```python
from build123d import *

# Parameters (mm, degrees)
BOSS_EXTRUDE1_DEPTH = 38.1


with BuildPart() as part:
    # Sketch1 → Boss-Extrude1 (new body)
    # profile 1 of 2: a face of its own
    with BuildSketch(Plane(origin=(0, 0, 0), x_dir=(1, 0, 0), z_dir=(0, 1, 0))):
        Polygon((0, 254), (0, 274), (-60.8, 250.891892714), (-60.8, 184.972107286), (-15, 175.951549331), (-15, 127), (0, 127), (0, 183.18932995), (-50.8, 193.194664975), (-50.8, 243.994664975), align=None)
    # profile 2 of 2: a face of its own
    with BuildSketch(Plane(origin=(0, 0, 0), x_dir=(1, 0, 0), z_dir=(0, 1, 0))):
        Polygon((99.289745962, 271.5), (107.95, 271.5), (107.95, 274), (0, 274), (0, 254), (107.95, 254), (107.95, 256.5), align=None)
        Polygon((85.629491924, 256.5), (94.289745962, 271.5), (102.95, 256.5), align=None, mode=Mode.SUBTRACT)
        Polygon((58.308983849, 256.5), (66.969237886, 271.5), (75.629491924, 256.5), align=None, mode=Mode.SUBTRACT)
        Polygon((89.289745962, 271.5), (80.629491924, 256.5), (71.969237886, 271.5), align=None, mode=Mode.SUBTRACT)
        Polygon((30.988475773, 256.5), (39.648729811, 271.5), (48.308983849, 256.5), align=None, mode=Mode.SUBTRACT)
        Polygon((61.969237886, 271.5), (53.308983849, 256.5), (44.648729811, 271.5), align=None, mode=Mode.SUBTRACT)
        Polygon((34.648729811, 271.5), (25.988475773, 256.5), (17.328221735, 271.5), align=None, mode=Mode.SUBTRACT)
        Polygon((12.328221735, 271.5), (20.988475773, 256.5), (3.667967697, 256.5), align=None, mode=Mode.SUBTRACT)
    extrude(amount=BOSS_EXTRUDE1_DEPTH)

    # Mirror1: part across plane


with BuildPart() as part_1:
    add(part.part)
    add(part.part.mirror(Plane(origin=(0, 38.1, -127), x_dir=(1, 0, 0), z_dir=(0, 0, -1))))

    # Mirror2: part across plane


with BuildPart() as part_2:
    add(part_1.part)
    add(part_1.part.mirror(Plane(origin=(107.95, 38.1, -254), x_dir=(0, 0, 1), z_dir=(-1, 0, 0))))


solid = part_2.part
```
Part model, mm, in its own coordinate system. A direction names the side the tool comes from. Coordinates: 2 decimals unless noted, no trailing zeros. Loops run counter-clockwise (first coordinate to the right, second up) from the corner with the lowest first, then second, coordinate; pieces in that order, holes last. Notation, with made-up numbers: (44, 51.5) - (91, 51.5) arc R6 cw to (91, 56.5) - close; hole circle Ø1 at (2, -34). An arc over 180 degrees is marked (long way). Write item = value, one per line. Start each with the question number.
Item 1: Cut at A-A, the plane z = -228.5. Give the cut face in (x, y).
Item 2: Cut at C-C, the plane z = -163. Give the cut face in (x, y).
Item 3: 3-axis set-ups, long thin cutter, end or side, ignore diameter. For faces 5 (the flat face through (194.181, 18.783, -263.895)), 6 (the flat face through (-30, 18.8, -262.6)): which of +Z, -Z, +X, -X, +Y, -Y reach the whole face in a straight line?
Item 4: Mould opens along X. For faces 1 (the flat face through (98.56, 18.78, -264.1)), 2 (the flat face through (240.94, 18.78, -188.12)), 3 (the flat face through (-15, 19, -126)), 4 (the flat face through (230.9, 19, -126)) say: released by +X, released by -X, zero draft, split by the parting line, or undercut.
Item 5: Flat gauge pins, fed straight in: pin 1 Ø19 at (y, z) = (25.5, -103) entering from +X; pin 2 Ø6 at (x, y) = (238.5, 12.5) entering from -Z. Where does each tip first touch, or does it go through?
Item 6: Cut at B-B, the plane x = -9. Give the cut face in (y, z), and give its area (3 significant figures).
Item 7: Cut at D-D, the plane y = 25. State how many separate pieces and enclosed holes the cut face has, and give its area (3 significant figures).
Item 8: Wall check: L1, parallel to X at y = 20, z = -105; L2, parallel to X at y = 22, z = -31; L3, parallel to Z at x = 105.5, y = 21. Give the ranges that are in metal, low to high. Write a range as from..to.
The answers:
q1.outline = (-60.8, 0) - (-50.8, 0) - (-50.8, 38.1) - (-60.8, 38.1) - close; (266.7, 0) - (276.7, 0) - (276.7, 38.1) - (266.7, 38.1) - close
q2.outline = (-15, 0) - (0, 0) - (0, 38.1) - (-15, 38.1) - close; (215.9, 0) - (230.9, 0) - (230.9, 38.1) - (215.9, 38.1) - close
q3.face_5 = +Y, -Y
q3.face_6 = -Z, -X, +Y, -Y
q4.face_1 = undercut
q4.face_2 = undercut
q4.face_3 = released by -X
q4.face_4 = released by +X
q5.pin_1 = 230.9
q5.pin_2 = -266.55
q6.outline = (0, -270.58) - (38.1, -270.58) - (38.1, -252.23) - (0, -252.23) - close; (0, -184.96) - (38.1, -184.96) - (38.1, -69.04) - (0, -69.04) - close; (0, -1.77) - (38.1, -1.77) - (38.1, 16.58) - (0, 16.58) - close
q6.area = 5,820 mm2
q7.separate_pieces = 1
q7.enclosed_holes = 31
q7.area = 15,500 mm2
q8.L1 = -15..0, 215.9..230.9
q8.L2 = -60.8..-50.8, 266.7..276.7
q8.L3 = -274..-271.5, -260.74..-254, 0..6.74, 17.5..20
